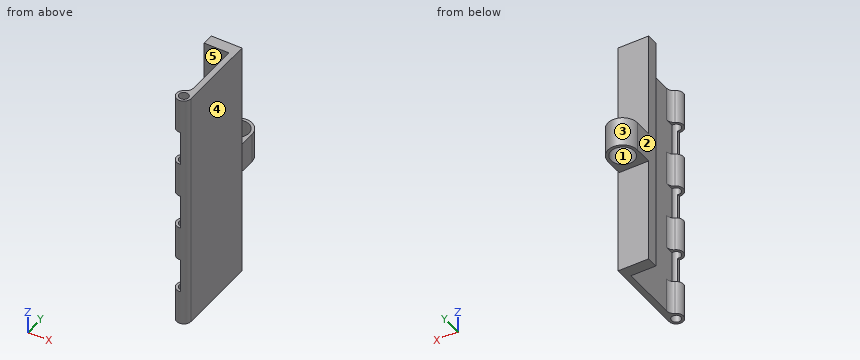
```python
from build123d import *

# Parameters (mm, degrees)
SKETCH1_R           = 1.5875
BOSS_EXTRUDE1_DEPTH = 82
SKETCH3_W           = 2
SKETCH3_H           = 82
BOSS_EXTRUDE4_DEPTH = 2.5
SKETCH6_W           = 82
SKETCH6_H           = 3.880734095
BOSS_EXTRUDE5_DEPTH = 8.39
BOSS_EXTRUDE6_START = -36
SKETCH8_R           = 4
BOSS_EXTRUDE6_DEPTH = 10
SKETCH10_W          = 11.720322
SKETCH10_H          = 6.929988864
CUT_EXTRUDE1_DEPTH  = 10
LPATTERN1_COUNT     = 3
LPATTERN1_PITCH     = 23.440644


with BuildPart() as part:
    # Sketch1 → Boss-Extrude1 (new body)
    with BuildSketch(Plane.XY):
        with BuildLine():
            Line((2.44, 0), (2.44, 25))
            Line((2.44, 25), (0.44, 25))
            Line((0.44, 25), (0.44, 4.489988864))
            ThreePointArc((0.44, 4.489988864), (0.044314057, 3.140225052), (-1.017489879, 2.217727293))
            ThreePointArc((-1.017489879, 2.217727293), (-1.317369481, -2.05381052), (2.44, 0))
        make_face()
        Circle(SKETCH1_R, mode=Mode.SUBTRACT)
    extrude(amount=BOSS_EXTRUDE1_DEPTH)

    # Sketch3 → Boss-Extrude4 (add)
    with BuildSketch(Plane(origin=(0, 25, 0), x_dir=(1, 0, 0), z_dir=(0, 1, 0))):
        with Locations((1.44, -41)):
            Rectangle(SKETCH3_W, SKETCH3_H)
    extrude(amount=BOSS_EXTRUDE4_DEPTH)

    # Sketch6 → Boss-Extrude5 (add)
    with BuildSketch(Plane.ZY.offset(-0.44)):
        with Locations((41, 25.559632953)):
            Rectangle(SKETCH6_W, SKETCH6_H)
    extrude(amount=BOSS_EXTRUDE5_DEPTH)

    # Sketch8 → Boss-Extrude6 (add)
    with BuildSketch(Plane(origin=(0, 0, 0), x_dir=(-1, 0, 0), z_dir=(0, 0, -1)).offset(BOSS_EXTRUDE6_START)):
        with BuildLine():
            Line((7.95, 27.5), (7.95, 33.5))
            ThreePointArc((7.95, 33.5), (2.95, 38.5), (-2.05, 33.5))
            Line((-2.05, 33.5), (-2.05, 27.5))
            Line((-2.05, 27.5), (7.95, 27.5))
        make_face()
        with Locations((2.95, 33.5)):
            Circle(SKETCH8_R, mode=Mode.SUBTRACT)
    extrude(amount=-BOSS_EXTRUDE6_DEPTH)

    # Sketch10 → Cut-Extrude1 (cut)
    with BuildSketch(Plane.ZY.offset(-0.44)):
        with Locations((17.580483, 1.024994432)):
            Rectangle(SKETCH10_W, SKETCH10_H)
    cut_extrude1 = extrude(amount=CUT_EXTRUDE1_DEPTH, mode=Mode.SUBTRACT)

    # LPattern1: Cut-Extrude1 ×3
    with Locations(*[(0, 0, i * LPATTERN1_PITCH) for i in range(1, LPATTERN1_COUNT)]):
        add(cut_extrude1, mode=Mode.SUBTRACT)


solid = part.part
```
Verification items for the finished model (mm, model axes). Face numbers are marked on the shaded views. A direction names the side the tool comes from. Give positions to 0.01 mm unless a question says otherwise; leave off trailing zeros. Loops run counter-clockwise (first coordinate to the right, second up) from the corner with the lowest first, then second, coordinate; pieces in that order, holes last. Notation, with made-up numbers: M -17,34 L 39,34 A17 ccw 39,67 Z; hole C -15,33 d11. An arc over 180 degrees is marked long. Return JSON: item names as keys, results as strings.
1) Tool access check on the marked faces 4 and 5. Record the directions out of +Z, -Z, +X, -X, +Y, -Y that give a thin tool (end or side, any length) a straight path to the whole face; none if there is none.
Findings:
{"face 4": "+Z, -Z, +X, +Y, -Y", "face 5": "+Z, -Z, -X"}
2) Material ranges on L1, parallel to Y at x = -6.5, z = 35; L2, parallel to Y at x = -0.25, z = 31.5; L3, parallel to Y at x = 0.75, z = 51, recorded low to high. Write a range as [from, to].
Findings:
{"L1": "y = [23.62, 27.5]", "L2": "y = [-2.43, -1.57], [1.57, 2.77], [23.62, 27.5]", "L3": "y = [-2.32, -1.4], [1.4, 27.5]"}
3) Section check C-C, the plane y = 14. Enter the section's corners in (x, z).
Findings:
{"outline": "M 0.44,0 L 2.44,0 L 2.44,82 L 0.44,82 Z"}
4) Section check A-A, the plane x = -3.25. Enter the section's corners in (y, z), and give its area (3 significant figures).
Findings:
{"outline": "M 23.62,0 L 27.5,0 L 27.5,36 L 29.51,36 L 29.51,46 L 27.5,46 L 27.5,82 L 23.62,82 Z; M 37.49,36 L 38.49,36 L 38.49,46 L 37.49,46 Z", "area": "348 mm2"}
5) Gauge pin test, flat ends, axial feed: P1, Ø2, axis at y = 6.5, z = 66.5, coming from the -X side; P2, Ø4, axis at x = -4, z = 31.5, coming from the -Y side; P3, Ø1.9, axis at x = 0, y = 0, coming from the +Z side. Record the tip position at first contact, or that the pin passes through.
Findings:
{"P1": "stops at x = 0.44", "P2": "stops at y = -1.4", "P3": "passes through"}
6) Mould release check, pull along Y, two halves, no side actions. Record for the marked faces 1, 2 and 3: released by +Y, released by -Y, zero draft, split by the parting line, or undercut.
Findings:
{"face 1": "undercut", "face 2": "zero draft", "face 3": "released by +Y"}
